from build123d import *

# Parameters (mm, degrees)
F1_DEPTH = 2400
F2_R     = 2
F3_R     = 1


with BuildPart() as f1:
    # F0 (on Top) → F1 (new body)
    with BuildSketch(Plane.XY):
        Polygon((20, 10), (-20, 10), (-20, -5), (-17, -5), (-17, 7), (-2, 7), (-2, -9.5), (-8.5, -9.5), (-8.5, -12.5), (0, -12.5), (8.5, -12.5), (8.5, -9.5), (2, -9.5), (2, 7), (17, 7), (17, -5), (20, -5), align=None)
    extrude(amount=F1_DEPTH)

    # F2
    f2_edges = [f1.edges().sort_by_distance(p)[0] for p in [
        (-20, 10, 1200),
        (20, 10, 1200),
    ]]
    fillet(f2_edges, radius=F2_R)

    # F3
    f3_edges = [f1.edges().sort_by_distance(p)[0] for p in [
        (-20, -5, 1200),
        (-17, -5, 1200),
        (-17, 7, 1200),
        (-8.5, -12.5, 1200),
        (8.5, -12.5, 1200),
        (8.5, -9.5, 1200),
        (2, 7, 1200),
        (17, -5, 1200),
        (20, -5, 1200),
        (17, 7, 1200),
        (-2, 7, 1200),
        (-8.5, -9.5, 1200),
        (-2, -9.5, 1200),
        (2, -9.5, 1200),
    ]]
    fillet(f3_edges, radius=F3_R)


solid = f1.part
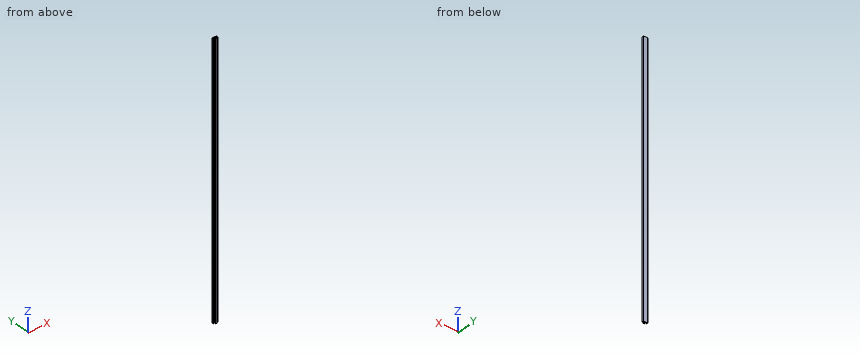
The model under review builds one solid part; all positions refer to its coordinate system, in mm. Give positions to 0.01 mm unless a question says otherwise; leave off trailing zeros. Loops run counter-clockwise (first coordinate to the right, second up) from the corner with the lowest first, then second, coordinate; pieces in that order, holes last. Notation, with made-up numbers: (85, 78) -> (108, 78) arc R14 cw to (108, 102) -> close; hole circle Ø4 at (71, 27.25). An arc over 180 degrees is marked (long way). Answer as a JSON object with one key per item and string values. Group by question number.
Q1. Take a section at A-A (y = 0.5). Write out the cut boundary in (x, z).
Q2. Insertion check: pin 1 (0.5 mm diameter, centred on x = 18.5, z = 776, fed in from -Y); pin 2 (8 mm diameter, centred on x = -7.5, y = -10, fed in from -Z); pin 3 (0.5 mm diameter, centred on y = -11, z = 600.5, fed in from -X); pin 4 (0.8 mm diameter, centred on y = -11, z = 1089.5, fed in from +X). Each pin has a flat end and moves straight along its axis. Give the tip position at first contact, or say it passes through.
Q3. Wall thickness on line 1 along X through (y, z) = (-2.5, 1720); line 2 along Y through (x, z) = (3.5, 215.5); line 3 along Y through (x, z) = (-11.5, 1769): over which ranges is each line inside the solid? List them lowest first.
Answer below:
{
 "1": {"outline": "(-20, 0) -> (-17, 0) -> (-17, 2400) -> (-20, 2400) -> close; (-2, 0) -> (2, 0) -> (2, 2400) -> (-2, 2400) -> close; (17, 0) -> (20, 0) -> (20, 2400) -> (17, 2400) -> close"},
 "2": {"pin 1": "stops at y = -5", "pin 2": "stops at z = 0", "pin 3": "stops at x = -8.5", "pin 4": "stops at x = 8.5"},
 "3": {"line 1": "x = -20 to -17, -2 to 2, 17 to 20", "line 2": "y = -12.5 to -9.5, 7 to 10", "line 3": "y = 7 to 10"}
}
